Model file for the job. Use its own axes, mm. A direction names the side the tool comes from. Coordinates: 2 decimals unless noted, no trailing zeros. Write each loop counter-clockwise with the first axis right and the second up, starting at its lowest first coordinate (ties: lowest second). Pieces come first, ordered by that corner, then holes. Notation, with made-up numbers: M 78,84 L 124,84 A14 ccw 124,109 Z; hole C 82,42 d5. An arc over 180 degrees is marked long. One line per question, with ' | ' between items. Start each with the question number.
(1) Wall check: probe 1 along Z at (x, y) = (16, 0.7); probe 2 along Z at (x, y) = (17.5, 1.75); probe 3 along Y at (x, z) = (-5, 16.25). Give the ranges that are in metal, low to high.
(2) Two-plate mould, pull along Z, no slides. Class faces 1 (the face through (-6.5, 1, 14)), 2 (the face through (5.2, 10.4, 0)), 3 (the face through (14.4, 1.5, 1.8)): +Z half, -Z half, draft (parallel to the pull), parting line (faces both ways), or undercut.
(3) Cut at B-B (x = 16). Write the cut outline in (y, z), plus the area to 3 significant figures.
(4) Cut at C-C (z = 3). Write the cut outline in (x, y).
(5) Tool access for faces 4 (the face through (12, 5, 9)), 5 (the face through (11, 1, 1)), 6 (the face through (-5.76, 1.479, 5.493)): list every direction of +Z, -Z, +X, -X, +Y, -Y with a clear straight run to the whole face (end or side of a thin tool).
(6) Cut at A-A (y = 2.25). Count the separate pieces of the cut face and the enclosed holes in it, plus the area to 3 significant figures.
(7) Flat gauge pins, fed straight in: pin 1 Ø3 at (y, z) = (8, 4) entering from +X; pin 2 Ø3 at (x, z) = (5, 11) entering from -Y; pin 3 Ø2.5 at (x, z) = (-4, 2) entering from +Y; pin 4 Ø3.5 at (x, y) = (-4, 2) entering from -Z. Where does each tip first touch, or does it go through?
from build123d import *

# Parameters (mm, degrees)
Y_KSEKLIK_EKSTR_ZYON1_DEPTH = 1
Y_KSEKLIK_EKSTR_ZYON2_DEPTH = 16
IZIM4_R                     = 2
Y_KSEKLIK_EKSTR_ZYON3_DEPTH = 3


with BuildPart() as part:
    # Çizim1 → Yükseklik-Ekstrüzyon1 (new body)
    with BuildSketch(Plane.XY):
        with BuildLine():
            Line((12, 1), (12, 9))
            ThreePointArc((12, 9), (11.707106781, 9.707106781), (11, 10))
            Line((11, 10), (1, 10))
            ThreePointArc((1, 10), (0.292893219, 9.707106781), (0, 9))
            Line((0, 9), (0, 1))
            ThreePointArc((0, 1), (0.292893219, 0.292893219), (1, 0))
            Line((1, 0), (-1.5, 0))
            Line((-1.5, 0), (-1.5, 8.5))
            ThreePointArc((-1.5, 8.5), (-0.621320344, 10.621320344), (1.5, 11.5))
            Line((1.5, 11.5), (10.5, 11.5))
            ThreePointArc((10.5, 11.5), (12.621320344, 10.621320344), (13.5, 8.5))
            Line((13.5, 8.5), (13.5, 0))
            Line((13.5, 0), (11, 0))
            ThreePointArc((11, 0), (11.707106781, 0.292893219), (12, 1))
        make_face()
    extrude(amount=Y_KSEKLIK_EKSTR_ZYON1_DEPTH)

    # Çizim3 → Yükseklik-Ekstrüzyon2 (add)
    with BuildSketch(Plane.XY.offset(1)):
        with BuildLine():
            Line((3, 0), (-1.5, 0))
            Line((-1.5, 0), (-1.5, 8.5))
            ThreePointArc((-1.5, 8.5), (-0.621320344, 10.621320344), (1.5, 11.5))
            Line((1.5, 11.5), (10.5, 11.5))
            ThreePointArc((10.5, 11.5), (12.621320344, 10.621320344), (13.5, 8.5))
            Line((13.5, 8.5), (13.5, 0))
            Line((13.5, 0), (9, 0))
            ThreePointArc((9, 0), (9.316227766, 0.051316702), (9.6, 0.2))
            ThreePointArc((9.6, 0.2), (12, 5), (9.6, 9.8))
            ThreePointArc((9.6, 9.8), (9.316227766, 9.948683298), (9, 10))
            Line((9, 10), (3, 10))
            ThreePointArc((3, 10), (2.683772234, 9.948683298), (2.4, 9.8))
            ThreePointArc((2.4, 9.8), (0, 5), (2.4, 0.2))
            ThreePointArc((2.4, 0.2), (2.683772234, 0.051316702), (3, 0))
        make_face()
    extrude(amount=Y_KSEKLIK_EKSTR_ZYON2_DEPTH)

    # Çizim4 → Yükseklik-Ekstrüzyon3 (add)
    with BuildSketch(Plane.XZ):
        Polygon((13.5, 0), (13.5, 6), (17, 6), (18.5, 5), (18.5, 1), (17, 0), align=None)
        with Locations((16, 3)):
            Circle(IZIM4_R, mode=Mode.SUBTRACT)
        Polygon((13.5, 17), (17, 17), (18.5, 16), (18.5, 12), (17, 11), (13.5, 11), align=None)
        with Locations((16, 14)):
            Circle(IZIM4_R, mode=Mode.SUBTRACT)
        Polygon((-1.5, 0), (-5, 0), (-6.5, 1), (-6.5, 5), (-5, 6), (-1.5, 6), align=None)
        with Locations((-4, 3)):
            Circle(IZIM4_R, mode=Mode.SUBTRACT)
        Polygon((-1.5, 17), (-1.5, 11), (-5, 11), (-6.5, 12), (-6.5, 16), (-5, 17), align=None)
        with Locations((-4, 14)):
            Circle(IZIM4_R, mode=Mode.SUBTRACT)
    extrude(amount=-Y_KSEKLIK_EKSTR_ZYON3_DEPTH)


solid = part.part
Filled in:
1) probe 1: 0 to 1, 5 to 6, 11 to 12, 16 to 17 | probe 2: 0.33 to 1.68, 4.32 to 5.67, 11.33 to 12.68, 15.32 to 16.67 | probe 3: 0 to 3
2) face 1: draft | face 2: -Z half | face 3: undercut
3) outline: M 0,0 L 3,0 L 3,1 L 0,1 Z; M 0,5 L 3,5 L 3,6 L 0,6 Z; M 0,11 L 3,11 L 3,12 L 0,12 Z; M 0,16 L 3,16 L 3,17 L 0,17 Z | area: 12.0 mm²
4) outline: M -6.5,0 L -6,0 L -6,3 L -6.5,3 Z; M -2,0 L 3,0 A1 cw 2.4,0.2 A6 cw 2.4,9.8 A1 cw 3,10 L 9,10 A1 cw 9.6,9.8 A6 cw 9.6,0.2 A1 cw 9,0 L 14,0 L 14,3 L 13.5,3 L 13.5,8.5 A3 ccw 10.5,11.5 L 1.5,11.5 A3 ccw -1.5,8.5 L -1.5,3 L -2,3 Z; M 18,0 L 18.5,0 L 18.5,3 L 18,3 Z
5) face 4: +Z, -Z | face 5: -Z | face 6: -X, +Y, -Y
6) separate pieces: 2 | enclosed holes: 4 | area: 136 mm²
7) pin 1: x = 13.5 | pin 2: y = 10 | pin 3: y = 3 | pin 4: z = 0
